```python
from build123d import *

# Parameters (mm, degrees)
BOX001002002_W           = 10
BOX001002002_H           = 22
BOX001002002_DEPTH       = 5
BOX001002_W              = 10
BOX001002_H              = 22
BOX001002_DEPTH          = 20
BOX001002_PITCH_ANGLE    = 44.999934
BOX001002001_W           = 10
BOX001002001_H           = 27
BOX001002001_DEPTH       = 22
BOX001002001_PITCH_ANGLE = 44.999934
BOX_W                    = 15
BOX_H                    = 25
BOX_DEPTH                = 15
BOX001001_W              = 15
BOX001001_H              = 10
BOX001001_DEPTH          = 1.5
BOX001_W                 = 15
BOX001_H                 = 10
BOX001_DEPTH             = 1.5


with BuildPart() as box005:
    # Box001002002 → Box001002002 (new body)
    with BuildSketch(Plane(origin=(-3, 1.5, -3), x_dir=(1, 0, 0), z_dir=(0, 0, 1))):
        with Locations((5, 11)):
            Rectangle(BOX001002002_W, BOX001002002_H)
    extrude(amount=BOX001002002_DEPTH)


with BuildPart() as box003:
    # Box001002 → Box001002 (new body)
    with BuildSketch(Plane.XY):
        with Locations((5, 11)):
            Rectangle(BOX001002_W, BOX001002_H)
    extrude(amount=BOX001002_DEPTH)


with BuildPart() as box003_1:
    # Box001002 pitch: moved
    add(box003.part.rotate(Axis((0, 0, 0), (0, 1, 0)), BOX001002_PITCH_ANGLE))


with BuildPart() as box003_2:
    # Box001002 placement: moved
    add(box003_1.part.moved(Location((1, 1.5, 0))))


with BuildPart() as fusion:
    # Box001002001 → Box001002001 (new body)
    with BuildSketch(Plane.XY):
        with Locations((5, 13.5)):
            Rectangle(BOX001002001_W, BOX001002001_H)
    extrude(amount=BOX001002001_DEPTH)


with BuildPart() as fusion_1:
    # Box001002001 pitch: moved
    add(fusion.part.rotate(Axis((0, 0, 0), (0, 1, 0)), BOX001002001_PITCH_ANGLE))


with BuildPart() as fusion_2:
    # Box001002001 placement: moved
    add(fusion_1.part.moved(Location((-8.71, -1, 7))))

    # Fusion: union Box005, Box003
    add(box005.part)
    add(box003_2.part)


with BuildPart() as cut:
    # Box → Box (new body)
    with BuildSketch(Plane.XY):
        with Locations((7.5, 12.5)):
            Rectangle(BOX_W, BOX_H)
    extrude(amount=BOX_DEPTH)

    # Cut: cut Fusion
    add(fusion_2.part, mode=Mode.SUBTRACT)


with BuildPart() as box002:
    # Box001001 → Box001001 (new body)
    with BuildSketch(Plane(origin=(0, -10, 0), x_dir=(1, 0, 0), z_dir=(0, 0, 1))):
        with Locations((7.5, 5)):
            Rectangle(BOX001001_W, BOX001001_H)
    extrude(amount=BOX001001_DEPTH)


with BuildPart() as mirrormount:
    # Box001 → Box001 (new body)
    with BuildSketch(Plane(origin=(0, 25, 0), x_dir=(1, 0, 0), z_dir=(0, 0, 1))):
        with Locations((7.5, 5)):
            Rectangle(BOX001_W, BOX001_H)
    extrude(amount=BOX001_DEPTH)

    # Fusion001: union Cut, Box002
    add(cut.part)
    add(box002.part)


solid = mirrormount.part
```
Part model, mm, in its own coordinate system. A direction names the side the tool comes from. Give positions to 0.01 mm unless a question says otherwise; leave off trailing zeros. Loops run counter-clockwise (first coordinate to the right, second up) from the corner with the lowest first, then second, coordinate; pieces in that order, holes last. Notation, with made-up numbers: M 86.5,-20 L 129.5,-20 A27 cw 129.5,11 Z; hole C 81,65 d7. An arc over 180 degrees is marked long. Return JSON: item names as keys, results as strings.
1) 3-axis set-ups, long thin cutter, end or side, ignore diameter. For faces 1 (the face through (14, 13, 15)), 2 (the face through (7, 30, 1.5)), 3 (the face through (2, 13, 2)), 4 (the face through (7, -5, 1.5)), 5 (the face through (9, 12, 8)): which of +Z, -Z, +X, -X, +Y, -Y reach the whole face in a straight line?
Calculated:
{"face 1": "+Z, +X, -X, +Y, -Y", "face 2": "+Z, +X, -X, +Y", "face 3": "-Z, +X, -X", "face 4": "+Z, +X, -X, -Y", "face 5": "-Z, +X"}
2) Saw through at B-B, the plane z = 5. List the corners of the cut face in (x, y), then the cut area to 3 significant figures.
Calculated:
{"outline": "M 3.43,0 L 15,0 L 15,1.5 L 6,1.5 L 6,23.5 L 15,23.5 L 15,25 L 3.43,25 Z", "area": "91.2 mm2"}
3) Pull direction Y, two halves, no side cores. Call faces 6 (the face through (7, 29, 0)), 7 (the face through (9, 25, 7)), 8 (the face through (11, 23.5, 4)), 9 (the face through (9, 0, 7)): released by +Y, released by -Y, zero draft, split by the parting line, or undercut.
Calculated:
{"face 6": "zero draft", "face 7": "released by +Y", "face 8": "undercut", "face 9": "released by -Y"}
4) Drill centre lines: line 1 (Y direction, x = 14, z = 2.75); line 2 (Z direction, x = 2.5, y = 28); line 3 (X direction, y = 10, z = 14). Where is each one in solid material? Low to high.
Calculated:
{"line 1": "y = 0 to 1.5, 23.5 to 25", "line 2": "z = 0 to 1.5", "line 3": "x = 12.43 to 15"}
5) Saw through at D-D, the plane z = 2.75. List the corners of the cut face in (x, y), then the cut area to 3 significant figures.
Calculated:
{"outline": "M 1.18,0 L 15,0 L 15,1.5 L 3.75,1.5 L 3.75,23.5 L 15,23.5 L 15,25 L 1.18,25 Z", "area": "97.9 mm2"}
6) Flat gauge pins, fed straight in: pin 1 Ø2 at (x, y) = (2.5, 11) entering from -Z; pin 2 Ø3 at (x, y) = (10.5, -4) entering from +Z; pin 3 Ø8 at (x, z) = (6, 11.5) entering from +Y. Where does each tip first touch, or does it go through?
Calculated:
{"pin 1": "stops at z = 2", "pin 2": "stops at z = 1.5", "pin 3": "stops at y = 25"}
7) Saw through at A-A, the plane y = 12.5. List the corners of the cut face in (x, z), then the cut area to 3 significant figures.
Calculated:
{"outline": "M 0.43,2 L 3,2 L 15,14 L 15,15 L 13.43,15 Z", "area": "32.9 mm2"}
8) Saw through at C-C, the plane x = 9.5. List the corners of the cut face in (y, z), then the cut area to 3 significant figures.
Calculated:
{"outline": "M -10,0 L 1.5,0 L 1.5,8.5 L 23.5,8.5 L 23.5,0 L 35,0 L 35,1.5 L 25,1.5 L 25,11.07 L 0,11.07 L 0,1.5 L -10,1.5 Z", "area": "120 mm2"}
